from build123d import *

# Parameters (mm, degrees)
F1_DEPTH = 8.75
F2_W     = 16.3845960051
F2_H     = 5.8396488756
F3_DEPTH = 10
F4_W     = 16.0876363516
F4_H     = 5.6553587645
F5_DEPTH = 10
F6_R     = 2.6324784905
F7_DEPTH = 25
F8_R     = 4
F9_DEPTH = 5
F10_R    = 2


# Not quite as in the source:
# - a feature names something its author has since deleted; it is built from what else it names


with BuildPart() as f1:
    # F0 (on Front) → F1 (new body, symmetric)
    with BuildSketch(Plane.XZ):
        Polygon((22.5, 19.5), (22.5, 29.5), (-22.5, 29.5), (-22.5, 19.5), (-33.2391485572, 19.5), (-44.5, 6.6135488451), (-44.5, -29.5), (-14, -29.5), (-17.5, -25.5), (17.5, -25.5), (14, -29.5), (44.5, -29.5), (44.5, 6.6135488451), (33.2391485572, 19.5), align=None)
    extrude(amount=F1_DEPTH, both=True)

    # F2 (on face) → F3 (cut)
    with BuildSketch(Plane.YZ.offset(44.5)):
        with Locations((0, 15.9833732828)):
            Rectangle(F2_W, F2_H)
        with Locations((0, 10.1437244073)):
            Rectangle(F2_W, F2_H)
    extrude(amount=-F3_DEPTH, mode=Mode.SUBTRACT)

    # F4 (on face) → F5 (cut)
    with BuildSketch(Plane(origin=(-44.5, 0, 0), x_dir=(0, -1, 0), z_dir=(-1, 0, 0))):
        with Locations((0, 15.8912282273)):
            Rectangle(F4_W, F4_H)
        with Locations((0, 10.2358694628)):
            Rectangle(F4_W, F4_H)
    extrude(amount=-F5_DEPTH, mode=Mode.SUBTRACT)

    # F6 (on face) → F7 (cut)
    with BuildSketch(Plane.XY.offset(19.5)):
        with BuildLine():
            ThreePointArc((-25.2370957881, -4.1691302322), (-26.0081308866, -2.3076868402), (-27.8695742786, -1.5366517417))
            Line((-27.8695742786, -1.5366517417), (-27.8695742786, -6.8016087227))
            ThreePointArc((-27.8695742786, -6.8016087227), (-26.0081308866, -6.0305736241), (-25.2370957881, -4.1691302322))
        make_face()
        with BuildLine():
            Line((-27.8695742786, -6.8016087227), (-27.8695742786, -1.5366517417))
            ThreePointArc((-27.8695742786, -1.5366517417), (-30.5020527691, -4.1691302322), (-27.8695742786, -6.8016087227))
        make_face()
        with BuildLine():
            Line((-27.8695742786, 1.5366517417), (-27.8695742786, 6.8016087227))
            ThreePointArc((-27.8695742786, 6.8016087227), (-30.5020527691, 4.1691302322), (-27.8695742786, 1.5366517417))
        make_face()
        with BuildLine():
            ThreePointArc((-25.2370957881, 4.1691302322), (-26.0081308866, 6.0305736241), (-27.8695742786, 6.8016087227))
            Line((-27.8695742786, 6.8016087227), (-27.8695742786, 1.5366517417))
            ThreePointArc((-27.8695742786, 1.5366517417), (-26.0081308866, 2.3076868402), (-25.2370957881, 4.1691302322))
        make_face()
        with Locations((-39.8695742786, 4.1691302322)):
            Circle(F6_R)
        with Locations((-39.8695742786, -4.1691302322)):
            Circle(F6_R)
        with Locations((27.8695742786, 4.1691302322)):
            Circle(F6_R)
        with Locations((27.8695742786, -4.1691302322)):
            Circle(F6_R)
        with Locations((39.8695742786, 4.1691302322)):
            Circle(F6_R)
        with Locations((39.8695742786, -4.1691302322)):
            Circle(F6_R)
    extrude(amount=-F7_DEPTH, mode=Mode.SUBTRACT)

    # F8 (on face) → F9 (join)
    with BuildSketch(Plane.XY.offset(29.5)):
        with Locations((7.5, 2.75)):
            Circle(F8_R)
    extrude(amount=F9_DEPTH)

    # F10
    f10_edges = [f1.edges().sort_by_distance(p)[0] for p in [
        (3.5, 2.75, 34.5),
    ]]
    fillet(f10_edges, radius=F10_R)


solid = f1.part
Could you check a few things on this model? Use its own coordinates, in mm. A direction names the side the tool comes from. Coordinates: 2 decimals unless noted, no trailing zeros. Order: outer loops, then holes, each group sorted by start corner. A loop starts at its lowest first (then second) coordinate and runs counter-clockwise, first axis right, second up. Notation, with made-up numbers: (-34, -3.75) -> (5, -3.75) arc R30 cw to (5, 33.25) -> close; hole circle Ø8 at (58.25, 55). An arc over 180 degrees is marked (long way). One line per item, written item: value. Start each with the question number.
1) Imagine slicing it at B-B on x = -2.5. List the corners of the cut face in (y, z) for me.
2) Imagine slicing it at A-A on z = 8.5. List the corners of the cut face in (x, y) for me, plus the area to 3 significant figures.
3) If I drill on L1, parallel to X at y = 2.25, z = 9.5; L2, parallel to X at y = -1.75, z = 5; L3, parallel to Y at x = 38, z = -0.5, over which ranges is the centre line in solid material (lowest first)? Write a range as [from, to].
4) We'd pull the mould along Z, two halves only. Please class faces 1 (the flat face through (-15.726, -0.123, -27.528)), 2 (the flat face through (28, 4, -5.5)), 3 (the cylindrical face through (4.326, 0.316, 30.979)): +Z half, -Z half, draft (parallel to the pull), parting line (faces both ways), or undercut.
5) Imagine slicing it at C-C on z = 23.5. List the corners of the cut face in (x, y) for me, plus the area to 4 significant figures.
6) I'm going to push flat-ended pins straight in: pin 1 (4 mm diameter, centred on x = 29, y = -5.5, fed in from +Z); pin 2 (5 mm diameter, centred on y = 3.5, z = 23, fed in from -X); pin 3 (1 mm diameter, centred on x = -4, y = -3.5, fed in from +Z). Where does each tip first touch, or does it pass through?
7) Which directions (+Z, -Z, +X, -X, +Y, -Y) give clear straight access to the entire face, cutting with the end or side of a thin tool? Please do faces 4 (the flat face through (28, 0, 19.5)), 5 (the flat face through (34.5, 0, 13)), 6 (the flat face through (-28, 0, 19.5)), 7 (the flat face through (-28, -4, -5.5)).
Answer list:
1. outline: (-8.75, -25.5) -> (8.75, -25.5) -> (8.75, 29.5) -> (-8.75, 29.5) -> close
2. outline: (-42.85, -8.75) -> (42.85, -8.75) -> (42.85, -8.19) -> (34.5, -8.19) -> (34.5, 8.19) -> (42.85, 8.19) -> (42.85, 8.75) -> (-42.85, 8.75) -> (-42.85, 8.04) -> (-34.5, 8.04) -> (-34.5, -8.04) -> (-42.85, -8.04) -> close; hole circle Ø5.26 at (-27.87, -4.17); hole circle Ø5.26 at (-27.87, 4.17); hole circle Ø5.26 at (27.87, -4.17); hole circle Ø5.26 at (27.87, 4.17)
2. area: 1,140 mm2
3. L1: x = [-34.5, -29.67], [-26.07, 26.07], [29.67, 34.5]
3. L2: x = [-44.5, -40.91], [-38.83, -28.91], [-26.83, 26.83], [28.91, 38.83], [40.91, 44.5]
3. L3: y = [-8.75, -6.02], [-2.32, 2.32], [6.02, 8.75]
4. face 1: undercut
4. face 2: +Z half
4. face 3: draft
5. outline: (-22.5, -8.75) -> (22.5, -8.75) -> (22.5, 8.75) -> (-22.5, 8.75) -> close
5. area: 787.5 mm2
6. pin 1: stops at z = 19.5
6. pin 2: stops at x = -22.5
6. pin 3: stops at z = 29.5
7. face 4: +Z, +X, +Y, -Y
7. face 5: +Z, +X
7. face 6: +Z, -X, +Y, -Y
7. face 7: +Z
